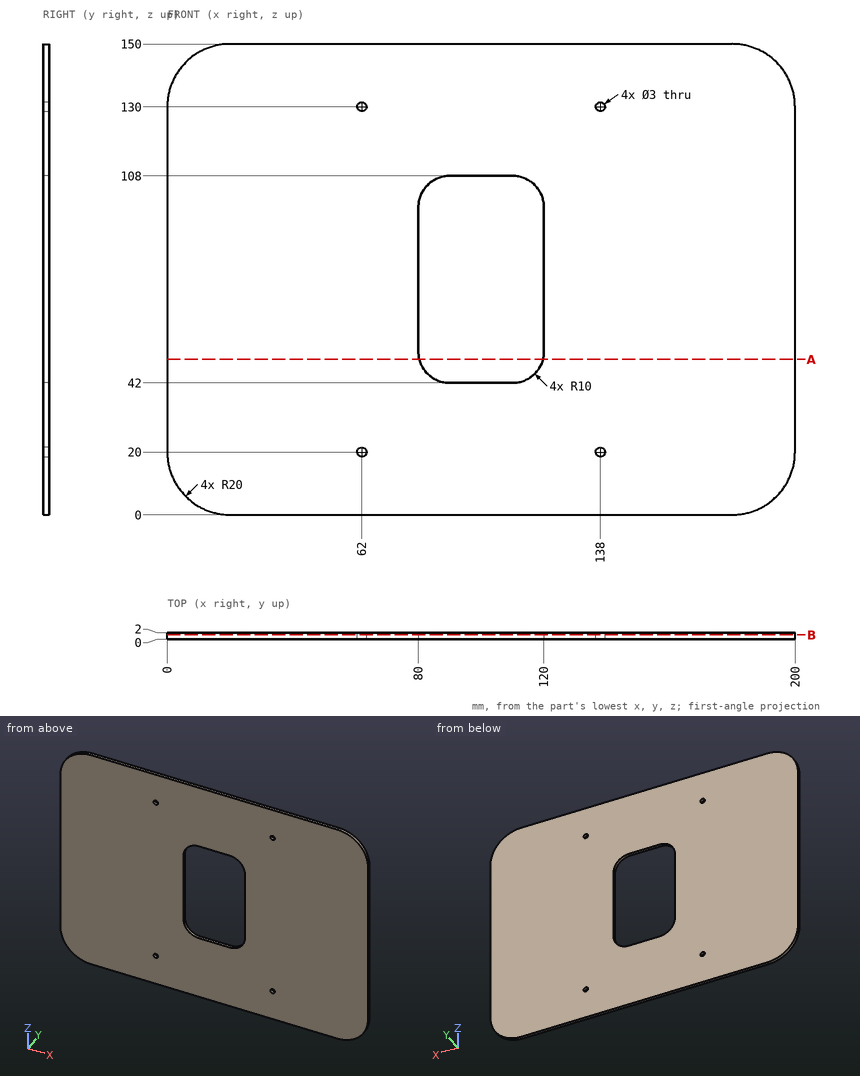
Could you check a few things on this drawing? It's one solid part, dimensions in mm from its lowest x, y, z. Give positions to 0.01 mm unless a question says otherwise; leave off trailing zeros. Order: outer loops, then holes, each group sorted by start corner. A loop starts at its lowest first (then second) coordinate and runs counter-clockwise, first axis right, second up. Notation, with made-up numbers: (61, 73) -> (80, 73) arc R38 ccw to (80, 112) -> close; hole circle Ø2 at (39, 53.25). An arc over 180 degrees is marked (long way). Use CSV: the item, a comma, the result in double quotes. Start each with the question number.
Item 1: If I drill on probe 1 along Z at (x, y) = (138, 1.4); probe 2 along X at (y, z) = (0.7, 20); probe 3 along X at (y, z) = (0.55, 92.5), over which ranges is the centre line in solid material (lowest first)? Write a range as [from, to].
Item 2: Suppose I cut it at B-B (y = 1.3). List the corners of the cut face in (x, z) for me.
Item 3: Suppose I cut it at A-A (z = 49.5). List the corners of the cut face in (x, y) for me.
Item 4: I'm going to push a flat-ended pin straight in: P1, Ø2.5, axis at x = 138, z = 20, coming from the -Y side. Where does the tip first touch, or does it pass through?
Answer block:
1,probe 1,"z = [0, 18.5], [21.5, 128.5], [131.5, 150]"
1,probe 2,"x = [0, 60.5], [63.5, 136.5], [139.5, 200]"
1,probe 3,"x = [0, 80], [120, 200]"
2,outline,"(0, 20) arc R20 ccw to (20, 0) -> (180, 0) arc R20 ccw to (200, 20) -> (200, 130) arc R20 ccw to (180, 150) -> (20, 150) arc R20 ccw to (0, 130) -> close; hole circle Ø3 at (62, 20); hole circle Ø3 at (62, 130); hole (80, 52) arc R10 ccw to (90, 42) -> (110, 42) arc R10 ccw to (120, 52) -> (120, 98) arc R10 ccw to (110, 108) -> (90, 108) arc R10 ccw to (80, 98) -> close; hole circle Ø3 at (138, 20); hole circle Ø3 at (138, 130)"
3,outline,"(0, 0) -> (80.32, 0) -> (80.32, 2) -> (0, 2) -> close; (119.68, 0) -> (200, 0) -> (200, 2) -> (119.68, 2) -> close"
4,P1,"passes through"
